from build123d import *

# Parameters (mm, degrees)
SKETCH1_W            = 80
SKETCH1_H            = 35
BOSS_EXTRUDE1_DEPTH  = 4
SKETCH2_R            = 14.775
CUT_EXTRUDE1_DEPTH   = 4
FILLET2_R            = 15
SKETCH3_W            = 12
SKETCH3_H            = 3.5
BOSS_EXTRUDE2_DEPTH  = 12
SKETCH4_R            = 2.75
CUT_EXTRUDE2_DEPTH   = 5
FILLET4_R            = 1
FILLET4_OF_MIRROR4_R = 1
FILLET5_R            = 15
SKETCH6_W            = 6.1
SKETCH6_H            = 2.250320618
SKETCH6_H_2          = 4.114705986
BOSS_EXTRUDE3_DEPTH  = 4


with BuildPart() as part:
    # Sketch1 → Boss-Extrude1 (new body)
    with BuildSketch(Plane.XY):
        Rectangle(SKETCH1_W, SKETCH1_H)
    extrude(amount=BOSS_EXTRUDE1_DEPTH)

    # Sketch2 → Cut-Extrude1 (cut)
    with BuildSketch(Plane.XY.offset(4)):
        with Locations((22.725, 0)):
            Circle(SKETCH2_R)
    cut_extrude1 = extrude(amount=-CUT_EXTRUDE1_DEPTH, mode=Mode.SUBTRACT)

    # Fillet2
    fillet2_edges = [part.edges().sort_by_distance(p)[0] for p in [
        (40, -17.5, 2),
        (-40, -17.5, 2),
    ]]
    fillet(fillet2_edges, radius=FILLET2_R)

    # Sketch3 → Boss-Extrude2 (add)
    with BuildSketch(Plane(origin=(0, 0, 0), x_dir=(-1, 0, 0), z_dir=(0, 0, -1))):
        with Locations((0, 15.75)):
            Rectangle(SKETCH3_W, SKETCH3_H)
    extrude(amount=BOSS_EXTRUDE2_DEPTH)

    # Sketch4 → Cut-Extrude2 (cut)
    with BuildSketch(Plane.XZ.offset(-14)):
        with Locations(Location((0, -6, 0), (0, 0, 270))):
            Circle(SKETCH4_R)
    extrude(amount=-CUT_EXTRUDE2_DEPTH, mode=Mode.SUBTRACT)

    # Fillet4
    fillet4_edges = [part.edges().sort_by_distance(p)[0] for p in [
        (7.95, 0, 0),
        (7.95, 0, 4),
    ]]
    fillet(fillet4_edges, radius=FILLET4_R)

    # Mirror4: Cut-Extrude1 across plane
    add(cut_extrude1.mirror(Plane(origin=(0, 0, 0), x_dir=(0, 0, 1), z_dir=(1, 0, 0))), mode=Mode.SUBTRACT)

    # Fillet4 of Mirror4
    fillet4_of_mirror4_edges = [part.edges().sort_by_distance(p)[0] for p in [
        (-7.95, 0, 0),
        (-7.95, 0, 4),
    ]]
    fillet(fillet4_of_mirror4_edges, radius=FILLET4_OF_MIRROR4_R)

    # Fillet5
    fillet5_edges = [part.edges().sort_by_distance(p)[0] for p in [
        (-40, 17.5, 2),
        (40, 17.5, 2),
    ]]
    fillet(fillet5_edges, radius=FILLET5_R)

    # Sketch6 → Boss-Extrude3 (add)
    with BuildSketch(Plane(origin=(0, 17.5, 0), x_dir=(1, 0, 0), z_dir=(0, 1, 0))):
        with Locations((0, 10.482941872)):
            Rectangle(SKETCH6_W, SKETCH6_H)
        with Locations((0, -0.375)):
            Rectangle(SKETCH6_W, SKETCH6_H_2)
    extrude(amount=BOSS_EXTRUDE3_DEPTH)


solid = part.part
Design review of the part built by this model. Coordinates are the model's own, in mm. A direction names the side the tool comes from. Coordinates: 2 decimals unless noted, no trailing zeros. Order: outer loops, then holes, each group sorted by start corner. A loop starts at its lowest first (then second) coordinate and runs counter-clockwise, first axis right, second up. Notation, with made-up numbers: M -28.75,-38.5 L 10.25,-38.5 A16 cw 10.25,-9.5 Z; hole C 37.25,60.5 d5. An arc over 180 degrees is marked long. Use a Markdown table: item, result.
(1) Add section C-C (y = 0). Give the boundary of the cut face in (x, z).
Worked answers:
| item | result |
|---|---|
| outline | M -40,0 L -38.5,0 A1 ccw -37.5,1 L -37.5,3 A1 ccw -38.5,4 L -40,4 Z; M -7.95,1 A1 ccw -6.95,0 L 6.95,0 A1 ccw 7.95,1 L 7.95,3 A1 ccw 6.95,4 L -6.95,4 A1 ccw -7.95,3 Z; M 37.5,1 A1 ccw 38.5,0 L 40,0 L 40,4 L 38.5,4 A1 ccw 37.5,3 Z |
(2) Add section D-D (y = 12). Count the separate pieces of the cut face and the enclosed holes in it, then the cut area to 3 significant figures.
Worked answers:
| item | result |
|---|---|
| separate pieces | 3 |
| enclosed holes | 0 |
| area | 152 mm2 |
(3) Wall thickness on probe 1 along X at (y, z) = (15.45, -6); probe 2 along X at (y, z) = (-13.5, 2); probe 3 along Z at (x, y) = (-35, -12.5): over which ranges is each line inside the solid? List them lowest first.
Worked answers:
| item | result |
|---|---|
| probe 1 | x = -6 to -2.75, 2.75 to 6 |
| probe 2 | x = -35.2 to -28.73, -16.72 to 16.72, 28.73 to 35.2 |
| probe 3 | z = 0 to 4 |
(4) Add section B-B (x = 0). Give the boundary of the cut face in (y, z).
Worked answers:
| item | result |
|---|---|
| outline | M -17.5,0 L 14,0 L 14,-3.25 L 17.5,-3.25 L 17.5,-1.68 L 21.5,-1.68 L 21.5,2.43 L 17.5,2.43 L 17.5,4 L -17.5,4 Z; M 14,-12 L 17.5,-12 L 17.5,-11.61 L 21.5,-11.61 L 21.5,-9.36 L 17.5,-9.36 L 17.5,-8.75 L 14,-8.75 Z |
(5) For P1, Ø6, axis at x = 1.5, z = -5.5, coming from the -Y side; P2, Ø4, axis at y = 16.5, z = -8, coming from the +X side; P3, Ø4.5, axis at x = -1, y = 18.5, coming from the -Z side; P4, Ø17.5, axis at x = 2, y = 4, coming from the -Z side, all flat-tipped, find the tip position at first contact; note any pin that passes through.
Worked answers:
| item | result |
|---|---|
| P1 | stops at y = 14 |
| P2 | stops at x = 6 |
| P3 | stops at z = -12 |
| P4 | stops at z = 0 |
(6) Add section A-A (z = -6). Give the boundary of the cut face in (x, y), then the cut area to 4 significant figures.
Worked answers:
| item | result |
|---|---|
| outline | M -6,14 L -2.75,14 L -2.75,17.5 L -6,17.5 Z; M 2.75,14 L 6,14 L 6,17.5 L 2.75,17.5 Z |
| area | 22.75 mm2 |
(7) Draft analysis for pull direction Z (two halves, no side actions). For faces 1 (the flat face through (-1, 0, 4)), 2 (the flat face through (0, -17.5, 2)), 3 (the flat face through (0, 19, -11.608)), 4 (the flat face through (0, 19, -1.682)), state which applies: released by +Z, released by -Z, zero draft, split by the parting line, or undercut.
Worked answers:
| item | result |
|---|---|
| face 1 | released by +Z |
| face 2 | zero draft |
| face 3 | released by -Z |
| face 4 | undercut |
(8) For faces 5 (the flat face through (0, 16, -12)), 6 (the flat face through (-3.05, 19, 0)), 7 (the flat face through (-6, 16, -6)), 8 (the flat face through (3.05, 19, -10)), list the 3-axis set-ups (+Z, -Z, +X, -X, +Y, -Y) from which the entire face can be reached by the end or side of a thin tool; tool diameter is ignored.
Worked answers:
| item | result |
|---|---|
| face 5 | -Z, +X, -X, +Y, -Y |
| face 6 | +Z, -Z, -X, +Y |
| face 7 | -Z, -X, +Y, -Y |
| face 8 | +Z, -Z, +X, +Y |
